Check sheet for the modelled part. Datum: model origin and axes. Units: mm. Round coordinates to 2 decimals unless told otherwise and drop trailing zeros. Write each loop counter-clockwise with the first axis right and the second up, starting at its lowest first coordinate (ties: lowest second). Pieces come first, ordered by that corner, then holes. Notation, with made-up numbers: (5.25, -1) -> (50.25, -1) arc R22 ccw to (50.25, 14) -> close; hole circle Ø10 at (47, 10). An arc over 180 degrees is marked (long way). Write item = value, one per line.
from build123d import *

# Parameters (mm, degrees)
BOSS_EXTRUDE1_DEPTH     = 31.75
CUT_EXTRUDE1_DEPTH      = 104.222934041
CUT_EXTRUDE1_DEPTH_BACK = 104.222934041
FILLET1_R               = 2.54


with BuildPart() as part:
    # Sketch1 → Boss-Extrude1 (new body)
    with BuildSketch(Plane(origin=(0, 0, 0), x_dir=(1, 0, 0), z_dir=(0, 1, 0))):
        with BuildLine():
            Line((-12.7, 73.846320133), (12.7, 73.846320133))
            Line((12.7, 73.846320133), (16.413720047, 95.436320133))
            ThreePointArc((16.413720047, 95.436320133), (0, 96.8375), (-16.413720047, 95.436320133))
            Line((-16.413720047, 95.436320133), (-12.7, 73.846320133))
        make_face()
    extrude(amount=BOSS_EXTRUDE1_DEPTH)

    # Sketch2 → Cut-Extrude1 (cut, two sides: drawn at the far end of the back side and taken through both)
    with BuildSketch(Plane(origin=(0, 0, 0), x_dir=(0, 0, -1), z_dir=(1, 0, 0)).offset(-CUT_EXTRUDE1_DEPTH_BACK)):
        Polygon((73.846320133, 30.48), (94.166320133, 0), (73.846320133, 0), align=None)
    extrude(amount=CUT_EXTRUDE1_DEPTH + CUT_EXTRUDE1_DEPTH_BACK, mode=Mode.SUBTRACT)

    # Fillet1
    # the kernel refuses this fillet: 2.54 mm, written as the material it takes off along each edge
    with BuildSketch(Plane(origin=(12.176698441, 35.043381397, -70.804065868), x_dir=(-0.9954788736987198, -0.07903081588642236, -0.05268721059094609), z_dir=(0.09498321967341544, -0.8282884898681249, -0.5521923265787502))) as fillet1_piece_1:
        with BuildLine():
            CenterArc((FILLET1_R * 0.867623718674, FILLET1_R), FILLET1_R, 188.108634364, 81.891365636)
            Line((-FILLET1_R * 0.122378694256, FILLET1_R * 0.858949575003), (0, 0))
            Line((0, 0), (FILLET1_R * 0.867623718674, 0))
        make_face()
    extrude(amount=47.817594086, mode=Mode.SUBTRACT)
    with BuildSketch(Plane(origin=(-16.718567485, -4.563381397, -97.208574398), x_dir=(-0.14041271821062315, 0.5603018628846251, -0.8163002456282387), z_dir=(0.09498321967341593, 0.8282884898681249, 0.5521923265787501))) as fillet1_piece_2:
        with BuildLine():
            CenterArc((FILLET1_R * 0.867623718674, -FILLET1_R), FILLET1_R, 90, 81.891365636)
            Line((-FILLET1_R * 0.122378694256, -FILLET1_R * 0.858949575003), (0, 0))
            Line((0, 0), (FILLET1_R * 0.867623718674, 0))
        make_face()
    extrude(amount=47.817594086, mode=Mode.SUBTRACT)
    with BuildSketch(Plane(origin=(19.593682793, 0, -94.166320133), x_dir=(0, 0, -1), z_dir=(-1, 0, 0))) as fillet1_piece_3:
        with BuildLine():
            CenterArc((FILLET1_R * 0.535183758488, -FILLET1_R), FILLET1_R, 90, 56.309932474)
            Line((-FILLET1_R * 0.29686653585, -FILLET1_R * 0.445299803775), (0, 0))
            Line((0, 0), (FILLET1_R * 0.535183758488, 0))
        make_face()
    extrude(amount=39.187365585, mode=Mode.SUBTRACT)
    with BuildSketch(Plane(origin=(-14.6226253, 30.48, -73.846320133), x_dir=(0, -0.8320502943378437, -0.5547001962252291), z_dir=(1, 0, 0))) as fillet1_piece_4:
        with BuildLine():
            CenterArc((FILLET1_R * 0.302775637732, FILLET1_R), FILLET1_R, 236.309932474, 33.690067526)
            Line((-FILLET1_R * 0.251924558493, FILLET1_R * 0.167949705662), (0, 0))
            Line((0, 0), (FILLET1_R * 0.302775637732, 0))
        make_face()
    extrude(amount=29.245250599, mode=Mode.SUBTRACT)


solid = part.part
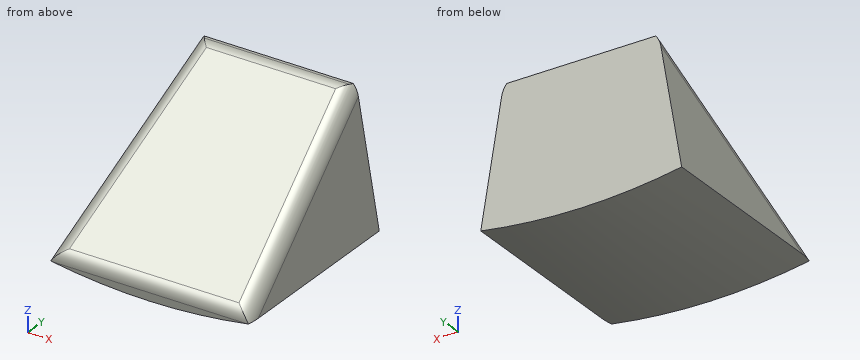
(1) Sectioned sample at A-A on x = 0. Enter the section's corners in (y, z).
Worked answers:
outline = (0, -96.84) -> (31.75, -96.84) -> (31.75, -73.85) -> (31.25, -73.85) arc R2.54 ccw to (29.84, -74.27) -> (1.13, -93.41) arc R2.54 ccw to (0, -95.53) -> close
(2) Material ranges on L1, parallel to X at y = 23.5, z = -94.5; L2, parallel to Y at x = -9, z = -87.5; L3, parallel to Z at x = -11, y = 9.5, recorded low to high. Write a range as [from, to].
Worked answers:
L1 = [-16.25, 16.25]
L2 = [10, 31.75]
L3 = [-96.21, -87.83]
(3) Sectioned sample at B-B on x = -8. Enter the section's corners in (y, z).
Worked answers:
outline = (0, -96.51) -> (31.75, -96.51) -> (31.75, -73.85) -> (31.25, -73.85) arc R2.54 ccw to (29.84, -74.27) -> (1.13, -93.41) arc R2.54 ccw to (0, -95.53) -> close
(4) Go/stop test with flat-tipped pins: P1, Ø1, axis at x = 8, y = 21.5, coming from the -Z side; P2, Ø12, axis at y = 13, z = -87, coming from the -X side; P3, Ø4, axis at x = -11.5, y = 16, coming from the -Z side; P4, Ø12, axis at x = 2.5, y = 25, coming from the -Z side. Record where each tip stops, or that it passes through.
Worked answers:
P1 = -96.55
P2 = -15.99
P3 = -96.37
P4 = -96.84
